Build history of the part. All positions in model axes, mm. Give positions to 0.01 mm unless a question says otherwise; leave off trailing zeros. Write each loop counter-clockwise with the first axis right and the second up, starting at its lowest first coordinate (ties: lowest second). Pieces come first, ordered by that corner, then holes. Notation, with made-up numbers: M 62,-37 L 95,-37 A23 cw 95,-18 Z; hole C -14,24.5 d8. An arc over 180 degrees is marked long. Return JSON: item names as keys, results as strings. Group by question number.
Q1. Band-saw the part on D-D, the plane x = -9.5. Give the cut face in (y, z).
Q2. Band-saw the part on B-B, the plane y = -3.25. Give the cut face in (x, z).
Q3. Wall check: probe 1 along Y at (x, z) = (-10.16, 0.85); probe 2 along X at (y, z) = (-2.25, 3); probe 3 along X at (y, z) = (-2, 0.6). Give the ranges that are in metal, low to high.
Q4. Band-saw the part on A-A, the plane x = 10.16. Give the cut face in (y, z), then the cut area to 3 significant figures.
Q5. Band-saw the part on C-C, the plane z = 2.7. Give the cut face in (x, y).
Autodesk Fusion 360 part; units mm, degrees
sketch "Sketch1" plane through (0, 0, 0) normal (0, 0, 1) x (1, 0, 0)
  line L0 (-12.7, 7.3182) -> (12.7, 7.3182)
  line L1 (12.7, 7.3182) -> (12.7, -5.3818)
  line L2 (12.7, -5.3818) -> (-12.7, -5.3818)
  line L3 (-12.7, -5.3818) -> (-12.7, 7.3182)
  circle A0 centre (-10.16, -2.8418) radius 1.1
  circle A1 centre (10.16, -2.8418) radius 1.1
  dimension "d1" = 25.4
  dimension "d2" = 12.7
  dimension "d3" = 2.2
  dimension "d4" = 2.2
  dimension "d5" = 20.32
  dimension "d6" = 2.54
  dimension "d7" = 2.54
  dimension "d8" = 2.54
extrude "Extrude1" add sketch "Sketch1" along normal blind 6.35
extrude "Extrude2" cut 1 faces at (3.1179, 4.1809, 6.35) along direction (0, 0, -1) blind 3.048
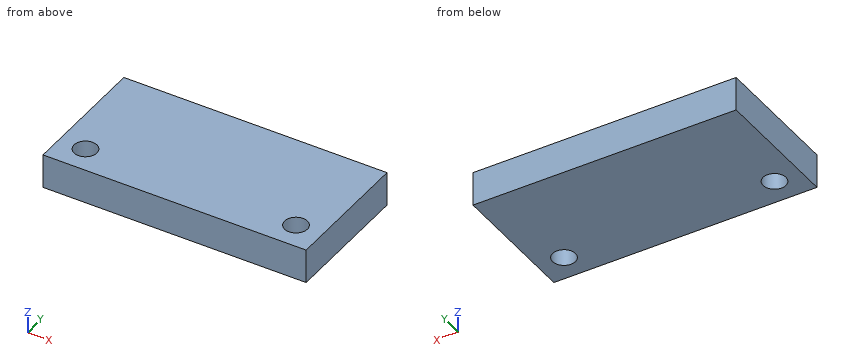
From the geometry:
{
 "1": {"outline": "M -5.38,0 L -3.72,0 L -3.72,3.3 L -5.38,3.3 Z; M -1.96,0 L 7.32,0 L 7.32,3.3 L -1.96,3.3 Z"},
 "2": {"outline": "M -12.7,0 L -11.18,0 L -11.18,3.3 L -12.7,3.3 Z; M -9.14,0 L 9.14,0 L 9.14,3.3 L -9.14,3.3 Z; M 11.18,0 L 12.7,0 L 12.7,3.3 L 11.18,3.3 Z"},
 "3": {"probe 1": "y = -5.38 to -3.94, -1.74 to 7.32", "probe 2": "x = -12.7 to -11.09, -9.23 to 9.23, 11.09 to 12.7", "probe 3": "x = -12.7 to -10.87, -9.45 to 9.45, 10.87 to 12.7"},
 "4": {"outline": "M -5.38,0 L -3.94,0 L -3.94,3.3 L -5.38,3.3 Z; M -1.74,0 L 7.32,0 L 7.32,3.3 L -1.74,3.3 Z", "area": "34.7 mm^2"},
 "5": {"outline": "M -12.7,-5.38 L 12.7,-5.38 L 12.7,7.32 L -12.7,7.32 Z; hole C -10.16,-2.84 d2.2; hole C 10.16,-2.84 d2.2"}
}
